Work out the finished part from the listing and answer in its coordinate system (mm). Face numbers are marked on the shaded views. A direction names the side the tool comes from. Round coordinates to 2 decimals unless told otherwise and drop trailing zeros. Loops run counter-clockwise (first coordinate to the right, second up) from the corner with the lowest first, then second, coordinate; pieces in that order, holes last. Notation, with made-up numbers: (-17.5, 81) - (0.5, 81) arc R18 ccw to (0.5, 103) - close; hole circle Ø9 at (37, -26). An arc over 180 degrees is marked (long way). Answer as CSV lines item,"result". Start each with the question number.
Q1. Section B-B on z = 0 is taken. Count the separate pieces of the cut face and the enclosed holes in it, then the cut area to 3 significant figures.
Q2. Straight lines are drawn through the part: L1, parallel to Y at x = -15.95, z = 0; L2, parallel to X at y = 17.75, z = 3.5; L3, parallel to Y at x = -13, z = -11. For each, find the intervals that lie inside material, in ascending order. Write a range as [from, to].
Q3. For the marked faces 4 and 5, determine the directions among +Z, -Z, +X, -X, +Y, -Y from which every point of the face is accessible in a straight line to the end or side of a thin tool.
Q4. Section D-D on y = 7.5 is taken. Write down the section's boundary in (x, z).
Q5. Section C-C on x = 6.5 is taken. Write down the section's boundary in (y, z) (3 decimals), then the cut area to 3 significant figures.
Q6. Each of these flat-tipped pins is pushed along its axis until it touches: pin 1 Ø3 at (x, y) = (15, 14) entering from -Z; pin 2 Ø4 at (y, z) = (16.45, -0.06) entering from -X; pin 3 Ø5 at (x, z) = (-2, 0) entering from +Y; pin 4 Ø2 at (x, z) = (-16, -7) entering from +Y. Where does it stop, or does it pass through?
Q7. Section A-A on y = 12.25 is taken. Write down the section's boundary in (x, z).
Q8. The mould has two halves that part along X. Classify the marked faces 1, 2 and 3: +X half, -X half, draft (parallel to the pull), parting line (faces both ways), or undercut.
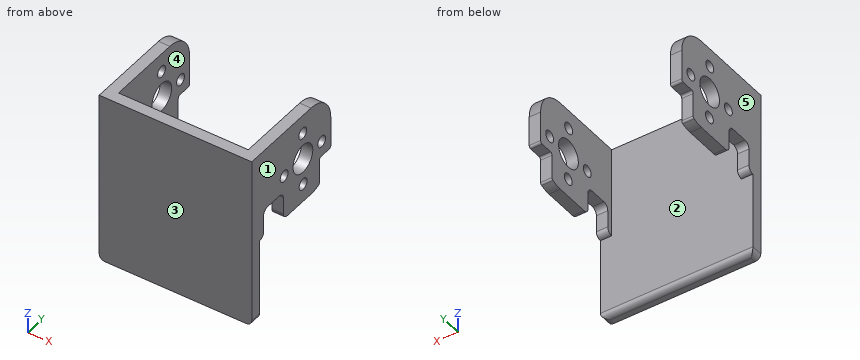
```python
from build123d import *

# Parameters (mm, degrees)
SKETCH1_W           = 34.036
SKETCH1_H           = 20.32
BOSS_EXTRUDE1_DEPTH = 25.4
SKETCH2_W           = 28.956
SKETCH2_H           = 20.32
CUT_EXTRUDE1_DEPTH  = 22.86
SKETCH3_R           = 1.27
SKETCH3_R_2         = 3.175
CUT_EXTRUDE2_DEPTH  = 44.667320687
FILLET2_R           = 6.35
SKETCH8_W           = 6.35
SKETCH8_H           = 6.35
CUT_EXTRUDE5_DEPTH  = 44.667320687
FILLET4_R           = 1.27
SKETCH10_W          = 8.835648684
SKETCH10_H          = 6.964146722
CUT_EXTRUDE6_DEPTH  = 44.667320687
FILLET6_R           = 0.508
FILLET7_R           = 0.508
SKETCH11_W          = 34.036
SKETCH11_H          = 2.54
BOSS_EXTRUDE3_DEPTH = 18.415
FILLET8_R           = 1.27


with BuildPart() as part:
    # Sketch1 → Boss-Extrude1 (new body)
    with BuildSketch(Plane(origin=(0, 0, 0), x_dir=(1, 0, 0), z_dir=(0, 1, 0))):
        Rectangle(SKETCH1_W, SKETCH1_H)
    extrude(amount=BOSS_EXTRUDE1_DEPTH)

    # Sketch2 → Cut-Extrude1 (cut)
    with BuildSketch(Plane(origin=(0, 25.4, 0), x_dir=(1, 0, 0), z_dir=(0, 1, 0))):
        Rectangle(SKETCH2_W, SKETCH2_H)
    extrude(amount=-CUT_EXTRUDE1_DEPTH, mode=Mode.SUBTRACT)

    # Sketch3 → Cut-Extrude2 (cut, through all)
    with BuildSketch(Plane.ZY.offset(17.018)):
        with Locations((0, 22.479)):
            Circle(SKETCH3_R)
        with Locations((-6.096, 16.51)):
            Circle(SKETCH3_R)
        with Locations((-0.127, 10.414)):
            Circle(SKETCH3_R)
        with Locations((5.969, 16.383)):
            Circle(SKETCH3_R)
        with Locations((-0.0635, 16.4465)):
            Circle(SKETCH3_R_2)
    extrude(amount=-CUT_EXTRUDE2_DEPTH, mode=Mode.SUBTRACT)

    # Fillet2
    fillet2_edges = [part.edges().sort_by_distance(p)[0] for p in [
        (-15.748, 25.4, -10.16),
        (15.748, 25.4, 10.16),
        (-15.748, 25.4, 10.16),
        (15.748, 25.4, -10.16),
    ]]
    fillet(fillet2_edges, radius=FILLET2_R)

    # Sketch8 → Cut-Extrude5 (cut, through all)
    with BuildSketch(Plane(origin=(17.018, 0, 0), x_dir=(0, 0, -1), z_dir=(1, 0, 0))):
        with Locations((6.985, 6.985)):
            Rectangle(SKETCH8_W, SKETCH8_H)
    extrude(amount=-CUT_EXTRUDE5_DEPTH, mode=Mode.SUBTRACT)

    # Fillet4
    fillet4_edges = [part.edges().sort_by_distance(p)[0] for p in [
        (15.748, 10.16, -10.16),
        (-15.748, 10.16, -10.16),
        (15.748, 3.81, -10.16),
        (-15.748, 3.81, -10.16),
        (15.748, 3.81, -3.81),
        (-15.748, 3.81, -3.81),
        (15.748, 10.16, -3.81),
        (-15.748, 10.16, -3.81),
    ]]
    fillet(fillet4_edges, radius=FILLET4_R)

    # Sketch10 → Cut-Extrude6 (cut, through all)
    with BuildSketch(Plane(origin=(17.018, 0, 0), x_dir=(0, 0, -1), z_dir=(1, 0, 0))):
        with Locations((7.840277159, 25.226914104)):
            Rectangle(SKETCH10_W, SKETCH10_H)
    extrude(amount=-CUT_EXTRUDE6_DEPTH, mode=Mode.SUBTRACT)

    # Fillet6
    fillet6_edges = [part.edges().sort_by_distance(p)[0] for p in [
        (15.748, 25.4, -3.422452817),
        (15.748, 21.744840743, -3.422452817),
        (15.748, 21.744840743, -9.559811594),
    ]]
    fillet(fillet6_edges, radius=FILLET6_R)

    # Fillet7
    fillet7_edges = [part.edges().sort_by_distance(p)[0] for p in [
        (-15.748, 21.744840743, -9.559811594),
        (-15.748, 25.4, -3.422452817),
        (-15.748, 21.744840743, -3.422452817),
    ]]
    fillet(fillet7_edges, radius=FILLET7_R)

    # Sketch11 → Boss-Extrude3 (add)
    with BuildSketch(Plane(origin=(0, 0, -10.16), x_dir=(-1, 0, 0), z_dir=(0, 0, -1))):
        with Locations((0, 1.27)):
            Rectangle(SKETCH11_W, SKETCH11_H)
    extrude(amount=BOSS_EXTRUDE3_DEPTH)

    # Fillet8
    fillet8_edges = [part.edges().sort_by_distance(p)[0] for p in [
        (17.018, 1.27, -28.575),
        (-17.018, 1.27, -28.575),
        (0, 2.54, -28.575),
    ]]
    fillet(fillet8_edges, radius=FILLET8_R)


solid = part.part
```
Findings:
1,separate pieces,"7"
1,enclosed holes,"0"
1,area,"145 mm^2"
2,L1,"y = [0, 9.15], [11.68, 13.27], [19.62, 21.21], [23.75, 25.4]"
2,L2,"x = [-17.02, -14.48], [14.48, 17.02]"
2,L3,"y = [0, 2.54]"
3,face 4,"+Z, -Z, +Y"
3,face 5,"+Z, -Z, -X, +Y, -Y"
4,outline,"(-17.02, -3.81) - (-14.48, -3.81) - (-14.48, 10.16) - (-17.02, 10.16) - close; (14.48, -3.81) - (17.02, -3.81) - (17.02, 10.16) - (14.48, 10.16) - close"
5,outline,"(0, -28.575) - (1.27, -28.575) arc R1.27 ccw to (2.54, -27.305) - (2.54, 10.16) - (0, 10.16) - close"
5,area,"98.0 mm^2"
6,pin 1,"stops at z = -10.16"
6,pin 2,"passes through"
6,pin 3,"stops at y = 2.54"
6,pin 4,"stops at y = 21.74"
7,outline,"(-17.02, -10.16) - (-14.48, -10.16) - (-14.48, 10.16) - (-17.02, 10.16) - close; (14.48, -10.16) - (17.02, -10.16) - (17.02, 10.16) - (14.48, 10.16) - close"
8,face 1,"+X half"
8,face 2,"undercut"
8,face 3,"draft"
